Here's how the part is built. I have some questions about the finished solid (model axes, mm). Face numbers are marked on the shaded views. A direction names the side the tool comes from. Give positions to 0.01 mm unless a question says otherwise; leave off trailing zeros. Loops run counter-clockwise (first coordinate to the right, second up) from the corner with the lowest first, then second, coordinate; pieces in that order, holes last. Notation, with made-up numbers: (76.25, -0.75) - (91.25, -0.75) arc R4 ccw to (91.25, 3.25) - close; hole circle Ø5 at (-27.75, 15.25). An arc over 180 degrees is marked (long way). Use one line per item in the form item = value.
from build123d import *

# Parameters (mm, degrees)
SKETCH1_R                 = 20
SKETCH1_R_2               = 16
BOSS_EXTRUDE1_DEPTH       = 10
SKETCH2_R                 = 1.75
BOSS_EXTRUDE2_DEPTH       = 3
BOSS_EXTRUDE2_2_DEPTH     = 3
BOSS_EXTRUDE3_OUTLINE_R   = 16
BOSS_EXTRUDE3_OUTLINE_R_2 = 12.5
BOSS_EXTRUDE3_DEPTH       = 58
FILLET1_R                 = 5
BOSS_EXTRUDE4_START       = 10
SKETCH3_R                 = 20
SKETCH3_R_2               = 14.5
BOSS_EXTRUDE4_DEPTH       = 10
CUT_EXTRUDE1_DEPTH        = 25
CUT_EXTRUDE2_DEPTH        = 3
BOSS_EXTRUDE5_START       = 48
SKETCH5_R                 = 20
SKETCH5_R_2               = 12.5
BOSS_EXTRUDE5_DEPTH       = 48
SKETCH6_R                 = 1.75
BOSS_EXTRUDE7_DEPTH       = 3
SKETCH7_R                 = 5
CUT_EXTRUDE3_DEPTH        = 3
CUT_EXTRUDE4_DEPTH        = 62.846584384
CUT_EXTRUDE4_DEPTH_BACK   = 62.846584384
SKETCH9_R                 = 1.75
BOSS_EXTRUDE8_START       = 10
SKETCH10_R                = 20
SKETCH10_R_2              = 18
BOSS_EXTRUDE8_DEPTH       = 10
FILLET5_R                 = 2
CUT_EXTRUDE5_START        = 39.893559
CUT_EXTRUDE5_DEPTH        = 10


# Read off the part's stored shape, not the designer's step: Boss-Extrude3
with BuildPart() as part:
    # Sketch1 → Boss-Extrude1 (new body)
    with BuildSketch(Plane(origin=(0, 0, 0), x_dir=(1, 0, 0), z_dir=(0, 1, 0))):
        with Locations(Location((0, 0, 0), (0, 0, 270))):
            Circle(SKETCH1_R)
        with Locations(Location((0, 0, 0), (0, 0, 270))):
            Circle(SKETCH1_R_2, mode=Mode.SUBTRACT)
    extrude(amount=BOSS_EXTRUDE1_DEPTH)



with BuildPart() as body_2:
    # Sketch2 → Boss-Extrude2 (new body)
    with BuildSketch(Plane(origin=(0, 0, 0), x_dir=(-1, 0, 0), z_dir=(0, -1, 0))):
        with BuildLine():
            Line((-9.387458609, 2), (-15.874507866, 2))
            ThreePointArc((-15.874507866, 2), (-16, 0), (-15.874507866, -2))
            Line((-15.874507866, -2), (-9.387458609, -2))
            ThreePointArc((-9.387458609, -2), (-4.75, 0), (-9.387458609, 2))
        make_face()
        with Locations(Location((-7.5, 0, 0), (0, 0, 90))):
            Circle(SKETCH2_R, mode=Mode.SUBTRACT)
    extrude(amount=BOSS_EXTRUDE2_DEPTH)


with BuildPart() as body_3:
    # Sketch2 → Boss-Extrude2 2 (new body)
    with BuildSketch(Plane(origin=(0, 0, 0), x_dir=(-1, 0, 0), z_dir=(0, -1, 0))):
        with BuildLine():
            Line((9.387458609, -2), (15.874507866, -2))
            ThreePointArc((15.874507866, -2), (16, 0), (15.874507866, 2))
            Line((15.874507866, 2), (9.387458609, 2))
            ThreePointArc((9.387458609, 2), (4.75, 0), (9.387458609, -2))
        make_face()
        with Locations(Location((7.5, 0, 0), (0, 0, 90))):
            Circle(SKETCH2_R, mode=Mode.SUBTRACT)
    extrude(amount=BOSS_EXTRUDE2_2_DEPTH)


    add(body_2.part)  # Boss-Extrude3 merges body 2
    # Boss-Extrude3 outline → Boss-Extrude3 (add)
    with BuildSketch(Plane(origin=(0, 0, 0), x_dir=(-1, 0, 0), z_dir=(0, -1, 0))):
        Circle(BOSS_EXTRUDE3_OUTLINE_R)
        Circle(BOSS_EXTRUDE3_OUTLINE_R_2, mode=Mode.SUBTRACT)
    extrude(amount=BOSS_EXTRUDE3_DEPTH)

    # Fillet1
    # the kernel refuses this fillet: 5 mm, written as the material it adds along each edge
    with BuildSketch(Plane(origin=(-12.338962679, -3, 2), x_dir=(0.44041013703938037, 0, 0.8977966981410402), z_dir=(0, 1, 0)), Plane(origin=(12.338962679, -3, -2), x_dir=(-0.4404101370393726, 0, -0.897796698141044), z_dir=(0, 1, 0))) as fillet1_piece_1:
        with BuildLine():
            CenterArc((5.821777357, 4.78348009), FILLET1_R, 205.259956012, 81.663200185)
            Line((1.299872312, 2.649850609), (1.209434211, 2.607178019))
            ThreePointArc((1.209434211, 2.607178019), (0.560156486, 1.368966318), (-0.08977967, 0.044041014))
            Line((-0.08977967, 0.044041014), (-0.029108887, -0.095669602))
            ThreePointArc((-0.029108887, -0.095669602), (3.638610848, -0.641299774), (7.306330583, -0.095669602))
            Line((7.306330583, -0.095669602), (7.277221696, 0))
        make_face()
    extrude(amount=3)
    with BuildSketch(Plane(origin=(-12.338962679, -3, -2), x_dir=(0.44041013703938064, 0, -0.8977966981410401), z_dir=(0, 1, 0)), Plane(origin=(12.338962679, -3, 2), x_dir=(-0.44041013703937265, 0, 0.8977966981410441), z_dir=(0, 1, 0))) as fillet1_piece_2:
        with BuildLine():
            CenterArc((5.821777357, -4.78348009), FILLET1_R, 73.076843803, 81.663200185)
            Line((1.299872312, -2.649850609), (1.209434211, -2.607178019))
            ThreePointArc((1.209434211, -2.607178019), (0.560156486, -1.368966318), (-0.08977967, -0.044041014))
            Line((-0.08977967, -0.044041014), (-0.029108887, 0.095669602))
            ThreePointArc((-0.029108887, 0.095669602), (3.638610848, 0.641299774), (7.306330583, 0.095669602))
            Line((7.306330583, 0.095669602), (7.277221696, 0))
        make_face()
    extrude(amount=3)


with BuildPart() as part_1:
    add(part.part)

    add(body_3.part)  # Boss-Extrude4 merges body 3
    # Sketch3 → Boss-Extrude4 (add)
    with BuildSketch(Plane(origin=(0, 0, 0), x_dir=(-1, 0, 0), z_dir=(0, -1, 0)).offset(BOSS_EXTRUDE4_START)):
        with Locations(Location((0, 0, 0), (0, 0, 90))):
            Circle(SKETCH3_R)
        Circle(SKETCH3_R_2, mode=Mode.SUBTRACT)
    extrude(amount=-BOSS_EXTRUDE4_DEPTH)

    # Sketch4 → Cut-Extrude1 (cut)
    with BuildSketch(Plane(origin=(0, 0, 0), x_dir=(1, 0, 0), z_dir=(0, 1, 0))):
        Polygon((-16.25, 3.175426481), (-19, 1.58771324), (-19, -1.58771324), (-16.25, -3.175426481), (-13.5, -1.58771324), (-13.5, 1.58771324), align=None)
        Polygon((16.25, 3.175426481), (13.5, 1.58771324), (13.5, -1.58771324), (16.25, -3.175426481), (19, -1.58771324), (19, 1.58771324), align=None)
    extrude(amount=CUT_EXTRUDE1_DEPTH, mode=Mode.SUBTRACT)

    # Sketch4<3> → Cut-Extrude2 (cut)
    with BuildSketch(Plane(origin=(0, 0, 0), x_dir=(1, 0, 0), z_dir=(0, 1, 0))):
        Polygon((-16.25, 3.175426481), (-19, 1.58771324), (-19, -1.58771324), (-16.25, -3.175426481), (-13.5, -1.58771324), (-13.5, 1.58771324), align=None)
        Polygon((16.25, 3.175426481), (13.5, 1.58771324), (13.5, -1.58771324), (16.25, -3.175426481), (19, -1.58771324), (19, 1.58771324), align=None)
    extrude(amount=-CUT_EXTRUDE2_DEPTH, mode=Mode.SUBTRACT)

    # Sketch5 → Boss-Extrude5 (add)
    with BuildSketch(Plane(origin=(0, -10, 0), x_dir=(-1, 0, 0), z_dir=(0, -1, 0)).offset(BOSS_EXTRUDE5_START)):
        with Locations(Location((0, 0, 0), (0, 0, 90))):
            Circle(SKETCH5_R)
        with Locations(Location((0, 0, 0), (0, 0, 223.053208616))):
            Circle(SKETCH5_R_2, mode=Mode.SUBTRACT)
    extrude(amount=-BOSS_EXTRUDE5_DEPTH)

    # Sketch6 → Boss-Extrude7 (add)
    # profile 1 of 3: a face of its own
    with BuildSketch(Plane(origin=(0, 0, 0), x_dir=(1, 0, 0), z_dir=(0, 1, 0))):
        with BuildLine():
            ThreePointArc((9.387458609, 2), (4.75, 0), (9.387458609, -2))
            ThreePointArc((9.387458609, -2), (10.476642124, -5.313902708), (9.134000475, -8.533465611))
            ThreePointArc((9.134000475, -8.533465611), (0, -12.5), (-9.134000475, -8.533465611))
            ThreePointArc((-9.134000475, -8.533465611), (-10.476642124, -5.313902708), (-9.387458609, -2))
            ThreePointArc((-9.387458609, -2), (-4.75, 0), (-9.387458609, 2))
            ThreePointArc((-9.387458609, 2), (-10.476642124, 5.313902708), (-9.134000475, 8.533465611))
            ThreePointArc((-9.134000475, 8.533465611), (0, 12.5), (9.134000475, 8.533465611))
            ThreePointArc((9.134000475, 8.533465611), (10.476642124, 5.313902708), (9.387458609, 2))
        make_face()
    # profile 2 of 3: a face of its own
    with BuildSketch(Plane(origin=(0, 0, 0), x_dir=(1, 0, 0), z_dir=(0, 1, 0))):
        with BuildLine():
            ThreePointArc((-9.387458609, 2), (-10.476642124, 5.313902708), (-9.134000475, 8.533465611))
            ThreePointArc((-9.134000475, 8.533465611), (-12.5, 0), (-9.134000475, -8.533465611))
            ThreePointArc((-9.134000475, -8.533465611), (-10.476642124, -5.313902708), (-9.387458609, -2))
            ThreePointArc((-9.387458609, -2), (-4.75, 0), (-9.387458609, 2))
        make_face()
        with Locations(Location((-7.5, 0, 0), (0, 0, 90))):
            Circle(SKETCH6_R, mode=Mode.SUBTRACT)
    # profile 3 of 3: a face of its own
    with BuildSketch(Plane(origin=(0, 0, 0), x_dir=(1, 0, 0), z_dir=(0, 1, 0))):
        with BuildLine():
            ThreePointArc((9.134000475, -8.533465611), (11.628091114, -4.586665132), (12.5, 0))
            ThreePointArc((12.5, 0), (11.628091114, 4.586665132), (9.134000475, 8.533465611))
            ThreePointArc((9.134000475, 8.533465611), (10.476642124, 5.313902708), (9.387458609, 2))
            ThreePointArc((9.387458609, 2), (4.75, 0), (9.387458609, -2))
            ThreePointArc((9.387458609, -2), (10.476642124, -5.313902708), (9.134000475, -8.533465611))
        make_face()
        with Locations(Location((7.5, 0, 0), (0, 0, 90))):
            Circle(SKETCH6_R, mode=Mode.SUBTRACT)
    extrude(amount=-BOSS_EXTRUDE7_DEPTH)

    # Sketch7 → Cut-Extrude3 (cut)
    with BuildSketch(Plane(origin=(0, 0, 0), x_dir=(1, 0, 0), z_dir=(0, 1, 0))):
        with Locations(Location((0, 0, 0), (0, 0, 270))):
            Circle(SKETCH7_R)
    extrude(amount=-CUT_EXTRUDE3_DEPTH, mode=Mode.SUBTRACT)

    # Sketch9 → Cut-Extrude4 (cut, two sides: drawn at the far end of the back side and taken through both)
    with BuildSketch(Plane(origin=(0, -3, 0), x_dir=(1, 0, 0), z_dir=(0, 1, 0)).offset(-CUT_EXTRUDE4_DEPTH_BACK)):
        with Locations(Location((-16.25, 0, 0), (0, 0, 270))):
            Circle(SKETCH9_R)
        with Locations(Location((16.25, 0, 0), (0, 0, 270))):
            Circle(SKETCH9_R)
    extrude(amount=CUT_EXTRUDE4_DEPTH + CUT_EXTRUDE4_DEPTH_BACK, mode=Mode.SUBTRACT)

    # Sketch10 → Boss-Extrude8 (add)
    with BuildSketch(Plane(origin=(0, -58, 0), x_dir=(-1, 0, 0), z_dir=(0, -1, 0)).offset(BOSS_EXTRUDE8_START)):
        with Locations(Location((0, 0, 0), (0, 0, 90))):
            Circle(SKETCH10_R)
        Circle(SKETCH10_R_2, mode=Mode.SUBTRACT)
    extrude(amount=-BOSS_EXTRUDE8_DEPTH)

    # Fillet5
    # the kernel refuses this fillet: 2 mm, written as the material it takes off along each edge
    with BuildSketch(Plane(origin=(7.5, 0, 0), x_dir=(0, 0, -1), z_dir=(-1, 0, 0))) as fillet5_piece_1:
        with BuildLine():
            CenterArc((1.75 + FILLET5_R, FILLET5_R), FILLET5_R, 180, 90)
            Line((1.75 + FILLET5_R, 0), (1.75, 0))
            Line((1.75, 0), (1.75, FILLET5_R))
        make_face()
    revolve(axis=Axis((7.5, 0, 0), (0, -1, 0)), mode=Mode.SUBTRACT)
    with BuildSketch(Plane(origin=(-7.5, 0, 0), x_dir=(0, 0, -1), z_dir=(-1, 0, 0))) as fillet5_piece_2:
        with BuildLine():
            CenterArc((1.75 + FILLET5_R, FILLET5_R), FILLET5_R, 180, 90)
            Line((1.75 + FILLET5_R, 0), (1.75, 0))
            Line((1.75, 0), (1.75, FILLET5_R))
        make_face()
    revolve(axis=Axis((-7.5, 0, 0), (0, -1, 0)), mode=Mode.SUBTRACT)

    # Sketch11 → Cut-Extrude5 (cut)
    with BuildSketch(Plane(origin=(0, -107.893559475, 0), x_dir=(1, 0, 0), z_dir=(0, 1, 0)).offset(CUT_EXTRUDE5_START)):
        Polygon((16.25, 3.175426481), (13.5, 1.58771324), (13.5, -1.58771324), (16.25, -3.175426481), (19, -1.58771324), (19, 1.58771324), align=None)
        Polygon((-16.25, 3.175426481), (-19, 1.58771324), (-19, -1.58771324), (-16.25, -3.175426481), (-13.5, -1.58771324), (-13.5, 1.58771324), align=None)
    extrude(amount=CUT_EXTRUDE5_DEPTH, mode=Mode.SUBTRACT)


solid = part_1.part
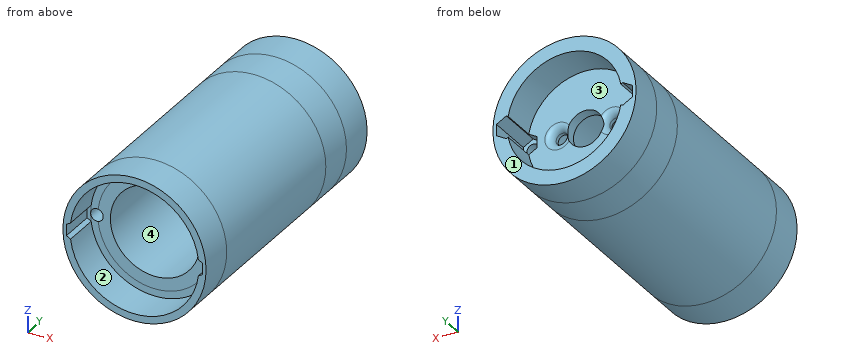
(1) If we section it at B-B (z = 11): List the corners of the cut face in (x, y) for me, plus the area to 3 significant figures.
Geometry says:
outline = (-16.7, -68) - (-14.25, -68) - (-14.25, -58) - (-5.94, -58) - (-5.94, -3) - (5.94, -3) - (5.94, -58) - (14.25, -58) - (14.25, -68) - (16.7, -68) - (16.7, 10) - (11.62, 10) - (11.62, 0) - (-11.62, 0) - (-11.62, 10) - (-16.7, 10) - close
area = 1,440 mm²
(2) For P1, Ø1, axis at x = 9, z = -10.5, coming from the -Y side; P2, Ø3, axis at x = -7.5, z = 0, coming from the -Y side; P3, Ø1.6, axis at y = -64, z = 0, coming from the -X side; P4, Ø8, axis at y = -6, z = -1, coming from the +X side, each with a flat end and sliding along its axis, tell me the tip position at first contact or that it passes through.
Geometry says:
P1 = -58
P2 = through
P3 = -20
P4 = 20
(3) If we section it at D-D (x = -7.5): List the corners of the cut face in (y, z) for me, plus the area to 3 significant figures.
Geometry says:
outline = (-68, -18.54) - (10, -18.54) - (10, -14.13) - (0, -14.13) - (0, -3.75) arc R2 ccw to (-2, -1.75) - (-3, -1.75) - (-3, -10) - (-58, -10) - (-58, -16.36) - (-68, -16.36) - close; (-68, 16.36) - (-58, 16.36) - (-58, 10) - (-3, 10) - (-3, 1.75) - (-2, 1.75) arc R2 ccw to (0, 3.75) - (0, 14.13) - (10, 14.13) - (10, 18.54) - (-68, 18.54) - close
area = 1,170 mm²
(4) For the marked faces 3 and 4, which set-ups out of +Z, -Z, +X, -X, +Y, -Y let a thin tool reach every point of the face, with its end or its side?
Geometry says:
face_3 = +Y
face_4 = -Y
(5) Thinking about a two-plate mould opening in Z: for the marked faces 1 and 2, which applies, pulls with the +Z half, pulls with the -Z half, needs draft (parallel to the pull), parting line crosses it, or undercut?
Geometry says:
face_1 = needs draft
face_2 = undercut
(6) If I drill on probe 1 along X at (y, z) = (-2.5, 0); probe 2 along X at (y, z) = (-42, 0); probe 3 along Z at (x, y) = (-0.5, -32.5), over which ranges is the centre line in solid material (lowest first)?
Geometry says:
probe_1 = -20 to -19, -13.5 to -9.25, -5.75 to -5, 5 to 5.75, 9.25 to 13.5, 19 to 20
probe_2 = -20 to -18, -14.5 to -12.5, 12.5 to 14.5, 18 to 20
probe_3 = -19.99 to -12.49, 12.49 to 19.99
(7) If we section it at A-A (x = 0): List the corners of the cut face in (y, z) for me, plus the area to 4 significant figures.
Geometry says:
outline = (-68, -20) - (10, -20) - (10, -16) - (0, -16) - (0, -5) - (-3, -5) - (-3, -12.5) - (-58, -12.5) - (-58, -18) - (-68, -18) - close; (-68, 18) - (-58, 18) - (-58, 12.5) - (-3, 12.5) - (-3, 5) - (0, 5) - (0, 16) - (10, 16) - (10, 20) - (-68, 20) - close
area = 1,035 mm²
(8) If we section it at C-C (y = -48): List the corners of the cut face in (x, z) for me, plus the area to 3 significant figures.
Geometry says:
outline = circle Ø40 at (0, 0); hole circle Ø3.5 at (-16.25, 0); hole circle Ø25 at (0, 0); hole circle Ø3.5 at (16.25, 0)
area = 747 mm²
